Could you check a few things on this drawing? It's one solid part, dimensions in mm from its lowest x, y, z. Round coordinates to 2 decimals unless told otherwise and drop trailing zeros. Loops run counter-clockwise (first coordinate to the right, second up) from the corner with the lowest first, then second, coordinate; pieces in that order, holes last. Notation, with made-up numbers: (26.25, 1.5) -> (37.25, 1.5) arc R12 cw to (37.25, 11.5) -> close; hole circle Ø8 at (-39.5, 7.25). An arc over 180 degrees is marked (long way). Put each result on its own line as item: value. Start each with the question number.
1. I'm going to push flat-ended pins straight in: P1, Ø0.6, axis at y = 1, z = 51, coming from the -X side; P2, Ø1, axis at x = 79.5, y = 1, coming from the +Z side; P3, Ø0.6, axis at x = 1.5, y = 0.5, coming from the -Z side. Where does each tip first touch, or does it pass through?
2. Imagine slicing it at A-A, the plane x = 29. Please give me the cut outline in (y, z), and give its area (3 significant figures).
3. Imagine slicing it at C-C, the plane y = 1. Count the separate pieces of the cut face and the enclosed holes in it, and give its area (3 significant figures).
4. Imagine slicing it at B-B, the plane z = 34.5. Please give me the cut outline in (x, y), and give its area (4 significant figures).
5. Imagine slicing it at D-D, the plane z = 9.5. Please give me the cut outline in (x, y), and give its area (3 significant figures).
6. I need wall thicknesses on line 1 (Z direction, x = 60, y = 1.9); line 2 (X direction, y = 1.8, z = 51); line 3 (X direction, y = 0.6, z = 28). Which ranges of each line are inside material? Lowest first, please. Write a range as [from, to].
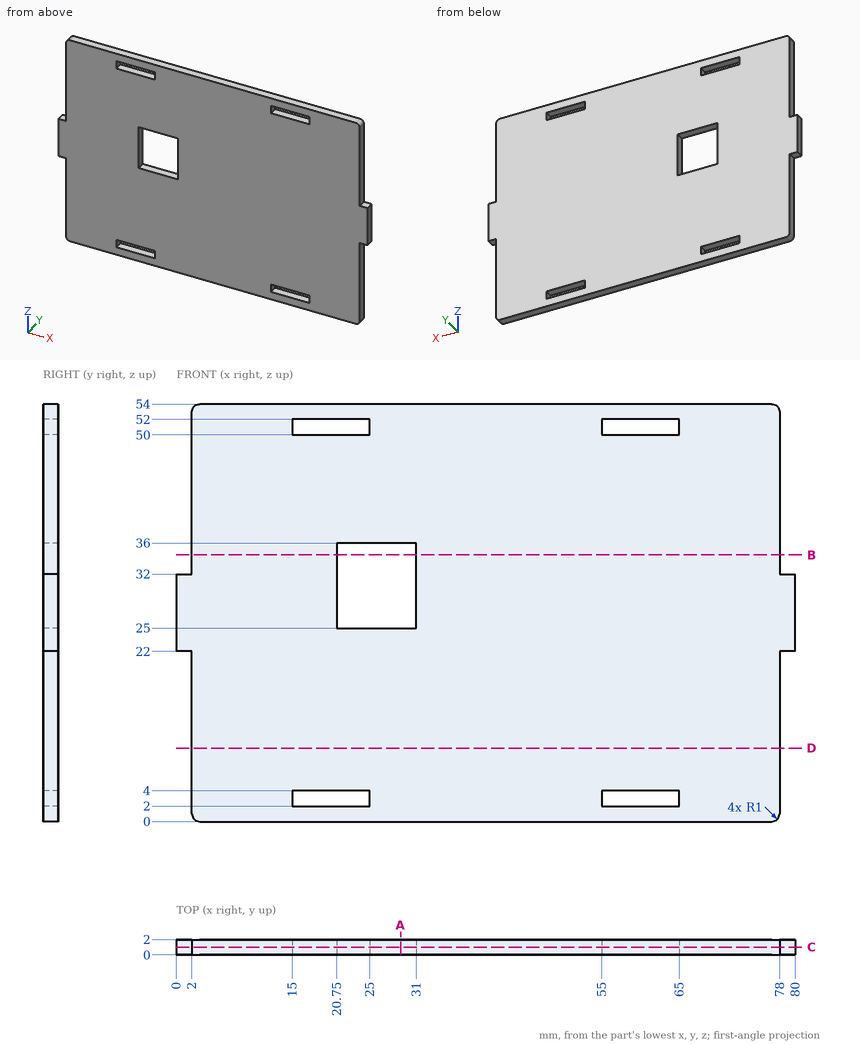
Entries:
1. P1: x = 2
1. P2: z = 32
1. P3: z = 22
2. outline: (0, 0) -> (2, 0) -> (2, 25) -> (0, 25) -> close; (0, 36) -> (2, 36) -> (2, 54) -> (0, 54) -> close
2. area: 86.0 mm^2
3. separate pieces: 1
3. enclosed holes: 5
3. area: 3,950 mm^2
4. outline: (2, 0) -> (20.75, 0) -> (20.75, 2) -> (2, 2) -> close; (31, 0) -> (78, 0) -> (78, 2) -> (31, 2) -> close
4. area: 131.5 mm^2
5. outline: (2, 0) -> (78, 0) -> (78, 2) -> (2, 2) -> close
5. area: 152 mm^2
6. line 1: [0, 2], [4, 50], [52, 54]
6. line 2: [2, 15], [25, 55], [65, 78]
6. line 3: [0, 20.75], [31, 80]
